Work out the finished part from the listing and answer in its coordinate system (mm). Face numbers are marked on the shaded views. A direction names the side the tool comes from. Round coordinates to 2 decimals unless told otherwise and drop trailing zeros. Write each loop counter-clockwise with the first axis right and the second up, starting at its lowest first coordinate (ties: lowest second). Pieces come first, ordered by that corner, then holes. Notation, with made-up numbers: (87.5, -4.5) -> (119.5, -4.5) arc R23 ccw to (119.5, 33.5) -> close; hole circle Ø10 at (-19.5, -29). An arc over 180 degrees is marked (long way). Answer as a JSON object with one key per item and string values. Group by question number.
from build123d import *

# Parameters (mm, degrees)
SKETCH2_R      = 10
EXTRUDE1_DEPTH = 16


with BuildPart() as part:
    # Sketch1 → Revolve1 (revolve)
    with BuildSketch(Plane(origin=(0, 0, 0), x_dir=(1, 0, 0), z_dir=(0, 1, 0))):
        with BuildLine():
            Line((-2.818193867, -7.327304055), (1.105880126, -7.327304055))
            Line((1.105880126, -7.327304055), (12.181806133, -7.327304055))
            Line((12.181806133, -7.327304055), (12.181806133, 6.672695945))
            ThreePointArc((12.181806133, 6.672695945), (11.888912914, 7.379802726), (11.181806133, 7.672695945))
            Line((11.181806133, 7.672695945), (8.181806133, 7.672695945))
            ThreePointArc((8.181806133, 7.672695945), (7.474699351, 7.965589164), (7.181806133, 8.672695945))
            Line((7.181806133, 8.672695945), (7.181806133, 16.172695945))
            ThreePointArc((7.181806133, 16.172695945), (6.449573086, 17.940462898), (4.681806133, 18.672695945))
            Line((4.681806133, 18.672695945), (-2.818193867, 18.672695945))
            Line((-2.818193867, 18.672695945), (-2.818193867, -7.327304055))
        make_face()
    revolve(axis=Axis((-2.818193867, 0, 7.327304055), (1, 0, 0)))

    # Sketch2 → Extrude1 (cut, through all)
    with BuildSketch(Plane(origin=(12.181806133, 0, 0), x_dir=(0, 0, -1), z_dir=(1, 0, 0))):
        with Locations((-7.327304055, 0)):
            Circle(SKETCH2_R)
    extrude(amount=-EXTRUDE1_DEPTH, mode=Mode.SUBTRACT)


solid = part.part
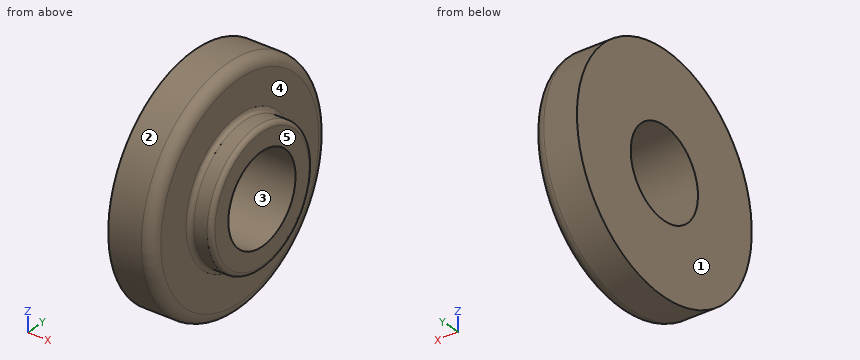
1) A cutting plane is placed at B-B on x = 10.5. Determine the outline of the cut face in (y, z).
2) Each of these flat-tipped pins is pushed along its axis until it touches: P1, Ø4, axis at y = 8, z = -11, coming from the +X side; P2, Ø6, axis at x = 1.5, z = 5, coming from the +Y side; P3, Ø8, axis at y = -2.5, z = 11.5, coming from the -X side; P4, Ø5, axis at x = 6.5, z = -13, coming from the -Y side. Where does it stop, or does it pass through?
3) For a pull along Y with two mould halves and no side action, classify the marked faces 1, 2 and 3 as released by +Y, released by -Y, zero draft, split by the parting line, or undercut.
4) A tool of negligible diameter and unlimited length cuts with its end or side. For the marked faces 4 and 5, from which of +Z, -Z, +X, -X, +Y, -Y can it reach the whole face along a straight path? Write none if from no direction.
5) A cutting plane is placed at A-A on y = 0. Determine the outline of the cut face in (x, z), plus the area to 3 significant figures.
6) Straight lines are drawn through the part: L1, parallel to X at y = -18, z = 2; L2, parallel to Y at x = 11.75, z = -0.5; L3, parallel to Y at x = -1.75, z = 11.5. For each, find the intervals that lie inside material, in ascending order.
Established:
{
 "1": {"outline": "circle Ø30 at (0, 7.33); hole circle Ø20 at (0, 7.33)"},
 "2": {"P1": "stops at x = 7.18", "P2": "stops at y = 26", "P3": "passes through", "P4": "stops at y = -18.54"},
 "3": {"face 1": "zero draft", "face 2": "split by the parting line", "face 3": "undercut"},
 "4": {"face 4": "+X", "face 5": "+Z, -Z, +X, +Y, -Y"},
 "5": {"outline": "(-2.82, -18.67) -> (4.68, -18.67) arc R2.5 ccw to (7.18, -16.17) -> (7.18, -8.67) arc R1 cw to (8.18, -7.67) -> (11.18, -7.67) arc R1 ccw to (12.18, -6.67) -> (12.18, -2.67) -> (-2.82, -2.67) -> close; (-2.82, 17.33) -> (12.18, 17.33) -> (12.18, 21.33) arc R1 ccw to (11.18, 22.33) -> (8.18, 22.33) arc R1 cw to (7.18, 23.33) -> (7.18, 30.83) arc R2.5 ccw to (4.68, 33.33) -> (-2.82, 33.33) -> close", "area": "367 mm²"},
 "6": {"L1": "x = -2.82 to 7.18", "L2": "y = -12.59 to -6.22, 6.22 to 12.59", "L3": "y = -25.66 to -9.09, 9.09 to 25.66"}
}
